from build123d import *

# Parameters (mm, degrees)
F1_DEPTH        = 19.05
F4_COPIES_COUNT = 4


# Not quite as in the source:
# - a pattern or mirror of a feature is missing from the dataset's text; its kind, count and spacing are read off the source's solid


with BuildPart() as f1:
    # F0 (on Top) → F1 (new body)
    with BuildSketch(Plane.XY):
        with BuildLine():
            ThreePointArc((10.71820488, -12.8734663491), (-11.8449578237, 11.8449578237), (12.8734663491, -10.71820488))
            Line((12.8734663491, -10.71820488), (15.0363144921, -12.8810530231))
            ThreePointArc((15.0363144921, -12.8810530231), (-14.0002192927, 14.0002192927), (12.8810530231, -15.0363144921))
            Line((12.8810530231, -15.0363144921), (10.71820488, -12.8734663491))
        make_face()
    extrude(amount=F1_DEPTH)

    # F4: sweep along a path in F3
    with BuildLine(Plane.YZ) as f4_path:
        Line((-32.4993, -25.4), (-19.7993, 0))
    # F2 (on face) → F4 (sweep)
    with BuildSketch(Plane(origin=(0, 0, 0), x_dir=(1, 0, 0), z_dir=(0, 0, -1))):
        with BuildLine():
            ThreePointArc((5.08, 19.136506486), (0, 19.7993), (-5.08, 19.136506486))
            Line((-5.08, 19.136506486), (-4.2979602309, 16.1905401251))
            ThreePointArc((-4.2979602309, 16.1905401251), (0, 16.7513), (4.2979602309, 16.1905401251))
            Line((4.2979602309, 16.1905401251), (5.08, 19.136506486))
        make_face()
    f4 = sweep(path=f4_path.line)

    # F4_copies: F4 ×4 about axis
    f4_copies_axis = Axis((0, 0, 0), (0, 0, 1))
    for i in range(1, F4_COPIES_COUNT):
        add(f4.rotate(f4_copies_axis, i * 360 / F4_COPIES_COUNT))

    # F7 (on Right) → F8 (revolve)
    with BuildSketch(Plane.YZ):
        Polygon((-18.7305401251, -38.1), (-28.8905401251, -25.4), (-31.836506486, -25.4), (-20.986948621, -38.9619473312), align=None)
    revolve(axis=Axis((0, 0, -16.1163), (0, 0, -1)))


solid = f1.part
For this review, take the finished solid that the model builds, in its own axes (mm). A direction names the side the tool comes from. Coordinates: 2 decimals unless noted, no trailing zeros. Write each loop counter-clockwise with the first axis right and the second up, starting at its lowest first coordinate (ties: lowest second). Pieces come first, ordered by that corner, then holes. Notation, with made-up numbers: (36, -8.75) -> (61, -8.75) arc R33 ccw to (61, 25.25) -> close; hole circle Ø11 at (12, -31.75). An arc over 180 degrees is marked (long way). Write each question's results on one line, items separated by ' | '. Start each with the question number.
1) Insertion check: pin 1 (1.5 mm diameter, centred on x = -18, z = 10, fed in from +Y); pin 2 (5 mm diameter, centred on x = 16.5, y = -7, fed in from -Z); pin 3 (0.8 mm diameter, centred on x = -32, y = -2, fed in from -Z). Each pin has a flat end and moves straight along its axis. Give the tip position at first contact, or say it passes through.
2) For faces 1 (the face through (24, 4.7, -12.6)), 2 (the face through (-4.7, 24, -12.6)), 3 (the face through (17.181, -8.936, -37.306)), 4 (the face through (-24, -4.7, -12.6)), list the 3-axis set-ups (+Z, -Z, +X, -X, +Y, -Y) from which the entire face can be reached by the end or side of a thin tool; tool diameter is ignored.
3) Wall thickness on L1, parallel to X at y = 0, z = 14; L2, parallel to Y at x = -2, z = -30: over which ranges is each line inside the solid? List them lowest first. Write a range as [from, to].
4) The part is to be moulded in two halves that separate along X. For faces 5 (the face through (-4.59, -24.08, -13.58)), 6 (the face through (-13.387, 14.588, 9.392)), 7 (the face through (13.94, -11.784, 9.392)), say which applies: +X half, -X half, draft (parallel to the pull), parting line (faces both ways), or undercut.
5) Consider section A-A (z = -20). Give the number of separate pieces and of enclosed holes in the cut face, plus the area to 3 significant figures.
6) Consider section C-C (z = -33). Write out the cut boundary in (x, y).
Geometry says:
1) pin 1: y = 9.72 | pin 2: z = -38.75 | pin 3: z = -25.62
2) face 1: +Y | face 2: -X | face 3: none | face 4: -Y
3) L1: [-19.8, -16.75], [16.75, 19.8] | L2: [-28.09, -25.13], [25.13, 28.09]
4) face 5: -X half | face 6: parting line | face 7: undercut
5) separate pieces: 4 | enclosed holes: 0 | area: 116 mm^2
6) outline: circle Ø51.51 at (0, 0); hole circle Ø45.62 at (0, 0)
